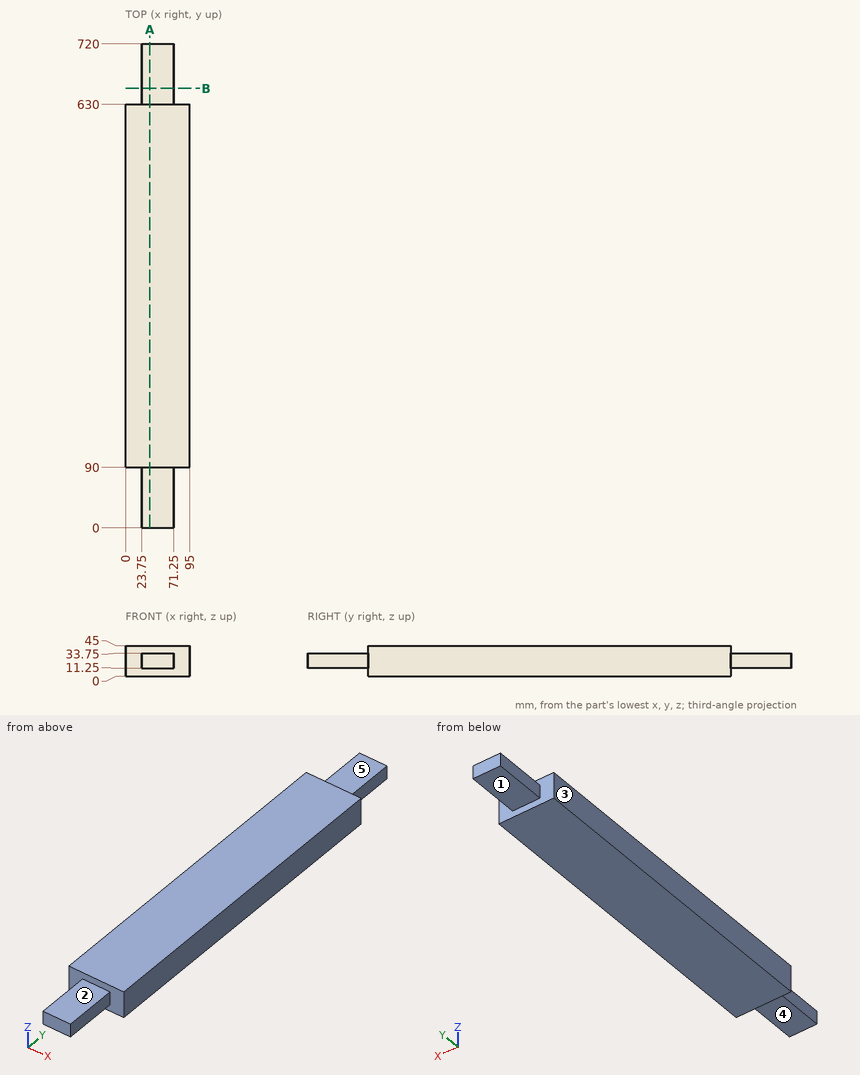
Geometry check sheet. Reference: drawing and pictorial views, mm from the part's lowest x, y, z. A direction names the side the tool comes from. Round coordinates to 2 decimals unless told otherwise and drop trailing zeros. Loops run counter-clockwise (first coordinate to the right, second up) from the corner with the lowest first, then second, coordinate; pieces in that order, holes last.
1. Sectioned sample at B-B on y = 654. Record the boundary of the cut face in (x, z).
2. Scan lines: probe 1 along Y at (x, z) = (76.5, 8); probe 2 along X at (y, z) = (680.5, 20); probe 3 along Z at (x, y) = (63.5, 60.5). Record each from-to range of solid material in increasing order.
3. Gauge pin test, flat ends, axial feed: pin 1 Ø25 at (y, z) = (673, 22) entering from +X; pin 2 Ø18 at (y, z) = (654.5, 25.5) entering from -X; pin 3 Ø24 at (x, y) = (51, 23.5) entering from -Z. Record the tip position at first contact, or that the pin passes through.
4. Set-up check for the marked faces 1, 2, 3, 4 and 5: record each of +Z, -Z, +X, -X, +Y, -Y from which the full face is reachable in a straight line by a thin tool's end or side.
5. Sectioned sample at A-A on x = 36. Record the boundary of the cut face in (y, z).
Recorded:
1. outline: (23.75, 11.25) - (71.25, 11.25) - (71.25, 33.75) - (23.75, 33.75) - close
2. probe 1: y = 90 to 630
2. probe 2: x = 23.75 to 71.25
2. probe 3: z = 11.25 to 33.75
3. pin 1: stops at x = 71.25
3. pin 2: stops at x = 23.75
3. pin 3: stops at z = 11.25
4. face 1: -Z, +X, -X, +Y
4. face 2: +Z, +X, -X, -Y
4. face 3: +Z, -Z, -X, +Y, -Y
4. face 4: -Z, +X, -X, -Y
4. face 5: +Z, +X, -X, +Y
5. outline: (0, 11.25) - (90, 11.25) - (90, 0) - (630, 0) - (630, 11.25) - (720, 11.25) - (720, 33.75) - (630, 33.75) - (630, 45) - (90, 45) - (90, 33.75) - (0, 33.75) - close
